Build history of the part. All positions in model axes, mm. Round coordinates to 2 decimals unless told otherwise and drop trailing zeros. Write each loop counter-clockwise with the first axis right and the second up, starting at its lowest first coordinate (ties: lowest second). Pieces come first, ordered by that corner, then holes.
Item 1: Band-saw the part on D-D, the plane z = -1.75. Count the separate pieces of the cut face and the enclosed holes in it, then the cut area to 3 significant figures.
Item 2: Band-saw the part on B-B, the plane z = 3.25. Write the cut outline in (x, y).
Item 3: Band-saw the part on A-A, the plane y = 37.5. Write the cut outline in (x, z).
Item 4: Wall check: probe 1 along Z at (x, y) = (11, -16); probe 2 along X at (y, z) = (3, -2.5); probe 3 along X at (y, z) = (3, -2.75). Give the ranges that are in metal, low to high.
Item 5: Mould opens along X. For faces 1 (the cylindrical face through (13.192, 10.91, -5.749)), 2 (the flat face through (26.3, 15.397, -5.013)), 3 (the cylindrical face through (-33.727, -25.861, 4.363)) say: +X half, -X half, draft (parallel to the pull), parting line (faces both ways), or undercut.
Item 6: Band-saw the part on C-C, the plane x = 0. Write the cut outline in (y, z), then the cut area to 3 significant figures.
Item 7: Drop flat-ended pins along their axis: pin 1 Ø5 at (y, z) = (-23, 1) entering from -X; pin 2 Ø1.5 at (y, z) = (3.5, -5.5) entering from +X; pin 3 Ø8 at (x, y) = (15, -2) entering from -Z; pin 4 Ø5 at (y, z) = (-2.5, -5.5) entering from -X. Give the stop position or say it passes through.
```python
from build123d import *

# Parameters (mm, degrees)
SKETCH1_R           = 42.5
BOSS_EXTRUDE1_DEPTH = 8.85
BOSS_EXTRUDE2_START = -10
SKETCH6_R           = 13.155696691
BOSS_EXTRUDE2_DEPTH = 10
CIRPATTERN1_COUNT   = 3


with BuildPart() as part:
    # Sketch1 → Boss-Extrude1 (new body)
    with BuildSketch(Plane.XY):
        Circle(SKETCH1_R)
    extrude(amount=BOSS_EXTRUDE1_DEPTH)

    # Sketch6 → Boss-Extrude2 (add)
    with BuildSketch(Plane(origin=(0, 1.664252335, 4.57249571), x_dir=(-1, 0, 0), z_dir=(0, 0.342020143, 0.939692621)).offset(BOSS_EXTRUDE2_START)):
        with Locations((0, 26.738166151)):
            Circle(SKETCH6_R)
    boss_extrude2 = extrude(amount=-BOSS_EXTRUDE2_DEPTH)

    # CirPattern1: Boss-Extrude2 ×3 about axis
    cirpattern1_axis = Axis((0, 0, 0), (0, 0, 1))
    for i in range(1, CIRPATTERN1_COUNT):
        add(boss_extrude2.rotate(cirpattern1_axis, i * 360 / CIRPATTERN1_COUNT))


solid = part.part
```
Results:
1. separate pieces: 3
1. enclosed holes: 0
1. area: 1,600 mm2
2. outline: circle Ø85 at (0, 0)
3. outline: (-20, 0) - (20, 0) - (20, 8.85) - (-20, 8.85) - close
4. probe 1: z = 0 to 8.85
4. probe 2: x = -31.48 to -18.08, 18.08 to 31.48
4. probe 3: x = -31.47 to -18.24, 18.24 to 31.47
5. face 1: undercut
5. face 2: +X half
5. face 3: parting line
6. outline: (-42.66, -0.58) - (-17.94, -9.58) - (-14.52, -0.18) - (-15.01, 0) - (42.5, 0) - (42.5, 8.85) - (-42.5, 8.85) - (-42.5, 0) - (-42.45, 0) - close
6. area: 894 mm2
7. pin 1: stops at x = -37.23
7. pin 2: stops at x = 33.18
7. pin 3: stops at z = 0
7. pin 4: passes through
